Source: CAD feature listing. Evaluate the final solid. Frame: model axes, mm. Round coordinates to 2 decimals unless told otherwise and drop trailing zeros. Order: outer loops, then holes, each group sorted by start corner. A loop starts at its lowest first (then second) coordinate and runs counter-clockwise, first axis right, second up. Notation, with made-up numbers: (-2, -23.75) -> (6, -23.75) arc R14 cw to (6, 3.25) -> close; hole circle Ø4 at (13, 8.5). An arc over 180 degrees is marked (long way). Answer as CSV lines item,"result". Start each with the question number.
(1) Contact query for a flat-ended pin moving along its axis: P1, Ø3, axis at y = -5, z = 69, coming from the -X side. Output: stop coordinate, or through.
(2) Line query: line 1 along X through (y, z) = (4, 54); line 2 along Y through (x, z) = (5.25, 86); line 3 along X through (y, z) = (-5.75, 160). Output: solid intervals per line, ascending. Write a range as from..to.
(3) Section query A-A (z = 232). Output: boundary loops of the cut face in (x, y), plus the area to 3 significant figures.
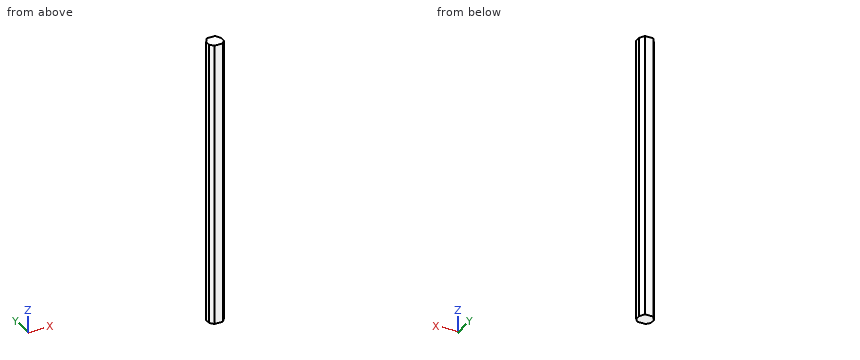
Autodesk Inventor part; units mm, degrees
ref_plane "YZ Plane" through (0, 0, 0) normal (1, 0, 0) x (0, 1, 0)
ref_plane "XZ Plane" through (0, 0, 0) normal (0, 1, 0) x (-1, 0, 0)
ref_plane "XY Plane" through (0, 0, 0) normal (0, 0, 1) x (1, 0, 0)
sketch "Sketch1" plane through (0, 0, 0) normal (0, 0, 1) x (1, 0, 0)
  line L0 (3.7307, 6.0592) -> (-3.572, 6.0592)
  line L1 (-3.572, 6.0592) -> (-6.5354, 1.4553)
  line L2 (-6.5354, 1.4553) -> (-6.5354, -3.2545)
  line L3 (-6.5354, -3.2545) -> (-3.572, -6.6413)
  line L4 (-3.572, -6.6413) -> (3.7307, -6.6413)
  line L5 (3.7307, 6.0592) -> (6.4435, 1.4553)
  line L6 (6.4435, 1.4553) -> (6.4435, -3.2545)
  line L7 (6.4435, -3.2545) -> (3.7307, -6.6413)
  point P0 (0, 0)
extrude "Extrusion1" add sketch "Sketch1" along normal blind 250
sketch "Sketch2" plane through (0, 0, 250) normal (0, 0, 1) x (1, 0, 0)
  point P0 (0, 0)
properties part number "pillar"
Answer block:
1,P1,"x = -6.32"
2,line 1,"-4.9..4.94"
2,line 2,"-4.74..3.48"
2,line 3,"-4.35..4.44"
3,outline,"(-6.54, -3.25) -> (-3.57, -6.64) -> (3.73, -6.64) -> (6.44, -3.25) -> (6.44, 1.46) -> (3.73, 6.06) -> (-3.57, 6.06) -> (-6.54, 1.46) -> close"
3,area,"142 mm2"
